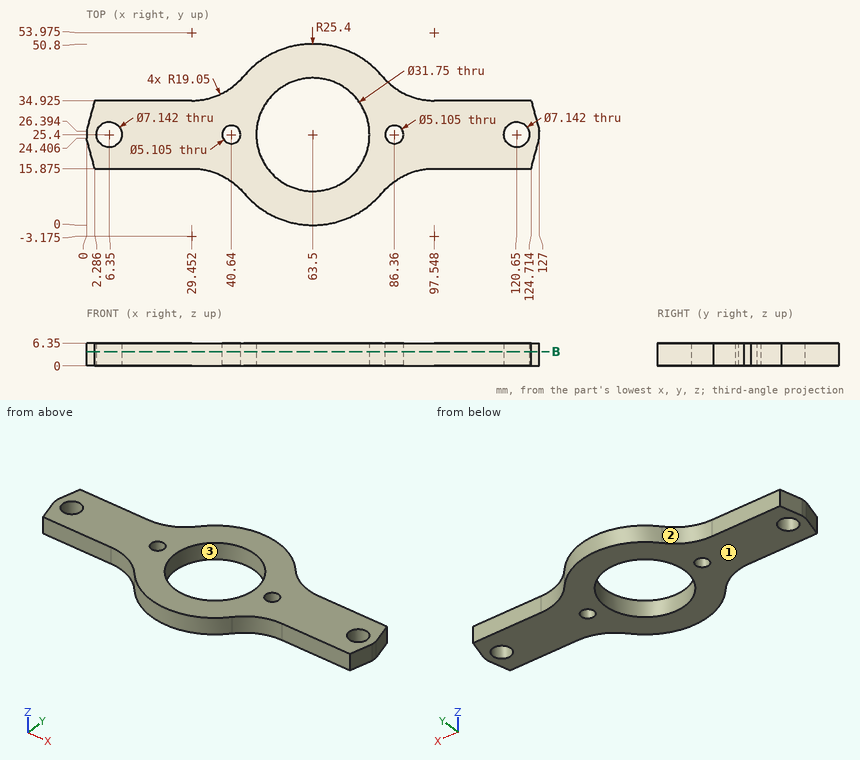
Can you work these out from the drawing? Everything is in mm from the part's minimum corner. Round coordinates to 2 decimals unless told otherwise and drop trailing zeros. Answer as CSV lines item,"result".
Item 1: Please list where these lines run through material, in increasing order: L1, parallel to Y at x = 63.5, z = 3.5 (1 decimal); L2, parallel to X at y = 22.5, z = 3 (1 decimal); L3, parallel to Y at x = 77.5, z = 2 (1 decimal). Write a range as [from, to].
From the geometry:
L1,"[0, 9.5], [41.3, 50.8]"
L2,"[0.5, 4.3], [8.4, 47.9], [79.1, 118.6], [122.7, 126.5]"
L3,"[4.2, 17.9], [32.9, 46.6]"
Item 2: We'd pull the mould along Y, two halves only. Please class the marked faces 1, 2 and 3: +Y half, -Y half, draft (parallel to the pull), parting line (faces both ways), or undercut.
From the geometry:
face 1,"draft"
face 2,"+Y half"
face 3,"undercut"
Item 3: Imagine slicing it at B-B on z = 4. Give the number of separate pieces and of enclosed holes in the cut face, and give its area (3 significant figures).
From the geometry:
separate pieces,"1"
enclosed holes,"5"
area,"2,610 mm2"
Item 4: For pin 1 (1.5 mm diameter, centred on x = 84, z = 2, fed in from -Y) (1 decimal); pin 2 (3 mm diameter, centred on x = 112, z = 1.5, fed in from +Y) (1 decimal); pin 3 (1 mm diameter, centred on x = 21, z = 4, fed in from -Y) (1 decimal), each with a flat end and sliding along its axis, tell me the tip position at first contact or that it passes through.
From the geometry:
pin 1,"y = 9.4"
pin 2,"y = 34.9"
pin 3,"y = 15.9"
